from build123d import *

# Parameters (mm, degrees)
SKETCH1_R           = 5.115
SKETCH1_R_2         = 4.75
BOSS_EXTRUDE1_DEPTH = 16
CUT_EXTRUDE1_DEPTH  = 96.686989711
SKETCH3_R           = 5.115
BOSS_EXTRUDE2_DEPTH = 16
BOSS_EXTRUDE3_DEPTH = 20


with BuildPart() as part:
    # Sketch1 → Boss-Extrude1 (new body)
    with BuildSketch(Plane.XY):
        with BuildLine():
            Line((-80, 3.444150891), (-76.699065455, 41.772249209))
            ThreePointArc((-76.699065455, 41.772249209), (-70.579654753, 49.5377007), (-61.024054334, 47))
            Line((-61.024054334, 47), (61.024054334, 47))
            ThreePointArc((61.024054334, 47), (70.579654753, 49.5377007), (76.699065455, 41.772249209))
            Line((76.699065455, 41.772249209), (80, 3.444150891))
            Line((80, 3.444150891), (80, -3.444150891))
            Line((80, -3.444150891), (75.129235099, -8.314915793))
            Line((75.129235099, -8.314915793), (68.240933316, -8.314915793))
            Line((68.240933316, -8.314915793), (63.370168415, -3.444150891))
            Line((63.370168415, -3.444150891), (63.370168415, -1.5))
            Line((63.370168415, -1.5), (-63.370168415, -1.5))
            Line((-63.370168415, -1.5), (-63.370168415, -3.444150891))
            Line((-63.370168415, -3.444150891), (-68.240933316, -8.314915793))
            Line((-68.240933316, -8.314915793), (-75.129235099, -8.314915793))
            Line((-75.129235099, -8.314915793), (-80, -3.444150891))
            Line((-80, -3.444150891), (-80, 3.444150891))
        make_face()
        with Locations((-71.685084207, 0)):
            Circle(SKETCH1_R, mode=Mode.SUBTRACT)
        with Locations((-67.732258267, 41)):
            Circle(SKETCH1_R_2, mode=Mode.SUBTRACT)
        with Locations(Location((67.732258267, 41, 0), (0, 0, 180))):
            Circle(SKETCH1_R_2, mode=Mode.SUBTRACT)
        with Locations(Location((71.685084207, 0, 0), (0, 0, 180))):
            Circle(SKETCH1_R, mode=Mode.SUBTRACT)
    extrude(amount=BOSS_EXTRUDE1_DEPTH)

    # Sketch2 → Cut-Extrude1 (cut, through all)
    with BuildSketch(Plane(origin=(0, 0, 0), x_dir=(-1, 0, 0), z_dir=(0, 0, -1))):
        with BuildLine():
            Line((-50.370168415, 3.5), (-50.370168415, -2.5))
            Line((-50.370168415, -2.5), (50.370168415, -2.5))
            Line((50.370168415, -2.5), (50.370168415, 3.5))
            ThreePointArc((50.370168415, 3.5), (50.955954852, 4.914213562), (52.370168415, 5.5))
            Line((52.370168415, 5.5), (57.370168415, 5.5))
            ThreePointArc((57.370168415, 5.5), (58.784381977, 6.085786438), (59.370168415, 7.5))
            Line((59.370168415, 7.5), (59.370168415, 12.5))
            ThreePointArc((59.370168415, 12.5), (58.784381977, 13.914213562), (57.370168415, 14.5))
            Line((57.370168415, 14.5), (52.370168415, 14.5))
            ThreePointArc((52.370168415, 14.5), (50.955954852, 15.085786438), (50.370168415, 16.5))
            Line((50.370168415, 16.5), (50.370168415, 21.795575149))
            ThreePointArc((50.370168415, 21.795575149), (49.892383898, 23.092826098), (48.687308391, 23.770270629))
            Line((48.687308391, 23.770270629), (25.72087261, 27.45872537))
            ThreePointArc((25.72087261, 27.45872537), (24.140212323, 27.648408909), (22.549472845, 27.711770579))
            Line((22.549472845, 27.711770579), (-22.549472845, 27.711770579))
            ThreePointArc((-22.549472845, 27.711770579), (-24.140212323, 27.648408909), (-25.72087261, 27.45872537))
            Line((-25.72087261, 27.45872537), (-48.687308391, 23.770270629))
            ThreePointArc((-48.687308391, 23.770270629), (-49.892383898, 23.092826098), (-50.370168415, 21.795575149))
            Line((-50.370168415, 21.795575149), (-50.370168415, 16.5))
            ThreePointArc((-50.370168415, 16.5), (-50.955954852, 15.085786438), (-52.370168415, 14.5))
            Line((-52.370168415, 14.5), (-57.370168415, 14.5))
            ThreePointArc((-57.370168415, 14.5), (-58.784381977, 13.914213562), (-59.370168415, 12.5))
            Line((-59.370168415, 12.5), (-59.370168415, 7.5))
            ThreePointArc((-59.370168415, 7.5), (-58.784381977, 6.085786438), (-57.370168415, 5.5))
            Line((-57.370168415, 5.5), (-52.370168415, 5.5))
            ThreePointArc((-52.370168415, 5.5), (-50.955954852, 4.914213562), (-50.370168415, 3.5))
        make_face()
    extrude(amount=-CUT_EXTRUDE1_DEPTH, mode=Mode.SUBTRACT)

    # Sketch3 → Boss-Extrude2 (add)
    with BuildSketch(Plane.XY.offset(16)):
        Polygon((-80, 3.444150891), (-80, -3.444150891), (-75.129235099, -8.314915793), (-68.240933316, -8.314915793), (-63.370168415, -3.444150891), (-63.370168415, 3.444150891), (-68.240933316, 8.314915793), (-75.129235099, 8.314915793), align=None)
        with Locations((-71.685084207, 0)):
            Circle(SKETCH3_R, mode=Mode.SUBTRACT)
    boss_extrude2 = extrude(amount=BOSS_EXTRUDE2_DEPTH)

    # Mirror1: Boss-Extrude2 across plane
    add(boss_extrude2.mirror(Plane(origin=(0, 0, 0), x_dir=(0, 0, 1), z_dir=(1, 0, 0))))

    # Sketch4 → Boss-Extrude3 (add)
    with BuildSketch(Plane.XY.offset(32)):
        with BuildLine():
            Line((-77.818836123, 28.770270629), (-43.370168415, 28.770270629))
            Line((-43.370168415, 28.770270629), (-43.370168415, 23.770270629))
            Line((-43.370168415, 23.770270629), (-48.687308391, 23.770270629))
            ThreePointArc((-48.687308391, 23.770270629), (-49.892383898, 23.092826098), (-50.370168415, 21.795575149))
            Line((-50.370168415, 21.795575149), (-50.370168415, 16.5))
            ThreePointArc((-50.370168415, 16.5), (-50.955954852, 15.085786438), (-52.370168415, 14.5))
            Line((-52.370168415, 14.5), (-57.370168415, 14.5))
            ThreePointArc((-57.370168415, 14.5), (-58.784381977, 13.914213562), (-59.370168415, 12.5))
            Line((-59.370168415, 12.5), (-59.370168415, 7.5))
            ThreePointArc((-59.370168415, 7.5), (-58.784381977, 6.085786438), (-57.370168415, 5.5))
            Line((-57.370168415, 5.5), (-52.370168415, 5.5))
            ThreePointArc((-52.370168415, 5.5), (-50.955954852, 4.914213562), (-50.370168415, 3.5))
            Line((-50.370168415, 3.5), (-50.370168415, -1.5))
            Line((-50.370168415, -1.5), (-63.370168415, -1.5))
            Line((-63.370168415, -1.5), (-63.370168415, -3.444150891))
            Line((-63.370168415, -3.444150891), (-68.240933316, -8.314915793))
            Line((-68.240933316, -8.314915793), (-75.129235099, -8.314915793))
            Line((-75.129235099, -8.314915793), (-80, -3.444150891))
            Line((-80, -3.444150891), (-80, 3.444150891))
            Line((-80, 3.444150891), (-77.818836123, 28.770270629))
        make_face()
    boss_extrude3 = extrude(amount=BOSS_EXTRUDE3_DEPTH)

    # Mirror2: Boss-Extrude3 across plane
    add(boss_extrude3.mirror(Plane(origin=(0, 0, 0), x_dir=(0, 0, 1), z_dir=(1, 0, 0))))


solid = part.part
Check sheet for the modelled part. Datum: model origin and axes. Units: mm. A direction names the side the tool comes from. Round coordinates to 2 decimals unless told otherwise and drop trailing zeros. Loops run counter-clockwise (first coordinate to the right, second up) from the corner with the lowest first, then second, coordinate; pieces in that order, holes last.
1. Set-up check for faces 4 (the flat face through (-63.37, -1, 26)), 5 (the flat face through (-55, 14.5, 8)), 6 (the cylindrical face through (-76.795, 0.225, 15.776)), 7 (the flat face through (50.37, 1, 42)), 8 (the flat face through (-43.37, 26, 42)): record each of +Z, -Z, +X, -X, +Y, -Y from which the full face is reachable in a straight line by a thin tool's end or side.
2. Scan lines: probe 1 along Z at (x, y) = (-70.5, 17.5); probe 2 along Y at (x, z) = (68.5, 12.5); probe 3 along Z at (x, y) = (-21, 35.5). Record each from-to range of solid material in increasing order.
3. Sectioned sample at B-B on y = 0. Record the boundary of the cut face in (x, z).
4. Gauge pin test, flat ends, axial feed: pin 1 Ø15.5 at (x, y) = (-18.5, 26) entering from +Z; pin 2 Ø8 at (x, z) = (9.5, 15) entering from -Y; pin 3 Ø1.5 at (x, z) = (-56, 37.5) entering from +Y; pin 4 Ø1 at (x, y) = (-55.5, 43) entering from -Z. Record the tip position at first contact, or that the pin passes through.
5. Sectioned sample at D-D on y = 19.5. Record the boundary of the cut face in (x, z), and give its area (3 significant figures).
6. Sectioned sample at A-A on z = 17.5. Record the boundary of the cut face in (x, y) (3 decimals), and give its area (3 significant figures).
7. Sectioned sample at C-C on y = 11. Record the boundary of the cut face in (x, z).
8. Mould release check, pull along X, two halves, no side actions. Record for faces 1 (the flat face through (72, 0, 32)), 2 (the flat face through (61, 28.77, 42)), 3 (the flat face through (77.531, 5.914, 23.888)): released by +X, released by -X, zero draft, split by the parting line, or undercut.
Recorded:
1. face 4: -Y
1. face 5: +Z, -Z
1. face 6: -Z
1. face 7: +Z, -Z, -Y
1. face 8: +Z, +Y, -Y
2. probe 1: z = 0 to 16, 32 to 52
2. probe 2: y = -8.31 to -4, 4 to 36.31, 45.69 to 49.97
2. probe 3: z = 0 to 16
3. outline: (-80, 0) - (-76.8, 0) - (-76.8, 32) - (-66.57, 32) - (-66.57, 0) - (-50.37, 0) - (-50.37, 16) - (-63.37, 16) - (-63.37, 32) - (-50.37, 32) - (-50.37, 52) - (-80, 52) - close; (50.37, 0) - (66.57, 0) - (66.57, 32) - (76.8, 32) - (76.8, 0) - (80, 0) - (80, 52) - (50.37, 52) - (50.37, 32) - (63.37, 32) - (63.37, 16) - (50.37, 16) - close
4. pin 1: stops at z = 16
4. pin 2: stops at y = 27.71
4. pin 3: stops at y = 28.77
4. pin 4: stops at z = 0
5. outline: (-78.62, 0) - (-50.37, 0) - (-50.37, 16) - (-78.62, 16) - close; (-78.62, 32) - (-50.37, 32) - (-50.37, 52) - (-78.62, 52) - close; (50.37, 0) - (78.62, 0) - (78.62, 16) - (50.37, 16) - close; (50.37, 32) - (78.62, 32) - (78.62, 52) - (50.37, 52) - close
5. area: 2,030 mm2
6. outline: (-80, -3.444) - (-75.129, -8.315) - (-68.241, -8.315) - (-63.37, -3.444) - (-63.37, 3.444) - (-68.241, 8.315) - (-75.129, 8.315) - (-80, 3.444) - close; (63.37, -3.444) - (68.241, -8.315) - (75.129, -8.315) - (80, -3.444) - (80, 3.444) - (75.129, 8.315) - (68.241, 8.315) - (63.37, 3.444) - close; hole circle Ø10.23 at (-71.685, 0); hole circle Ø10.23 at (71.685, 0)
6. area: 294 mm2
7. outline: (-79.35, 0) - (-59.37, 0) - (-59.37, 16) - (-79.35, 16) - close; (-79.35, 32) - (-59.37, 32) - (-59.37, 52) - (-79.35, 52) - close; (59.37, 0) - (79.35, 0) - (79.35, 16) - (59.37, 16) - close; (59.37, 32) - (79.35, 32) - (79.35, 52) - (59.37, 52) - close
8. face 1: undercut
8. face 2: zero draft
8. face 3: released by +X
